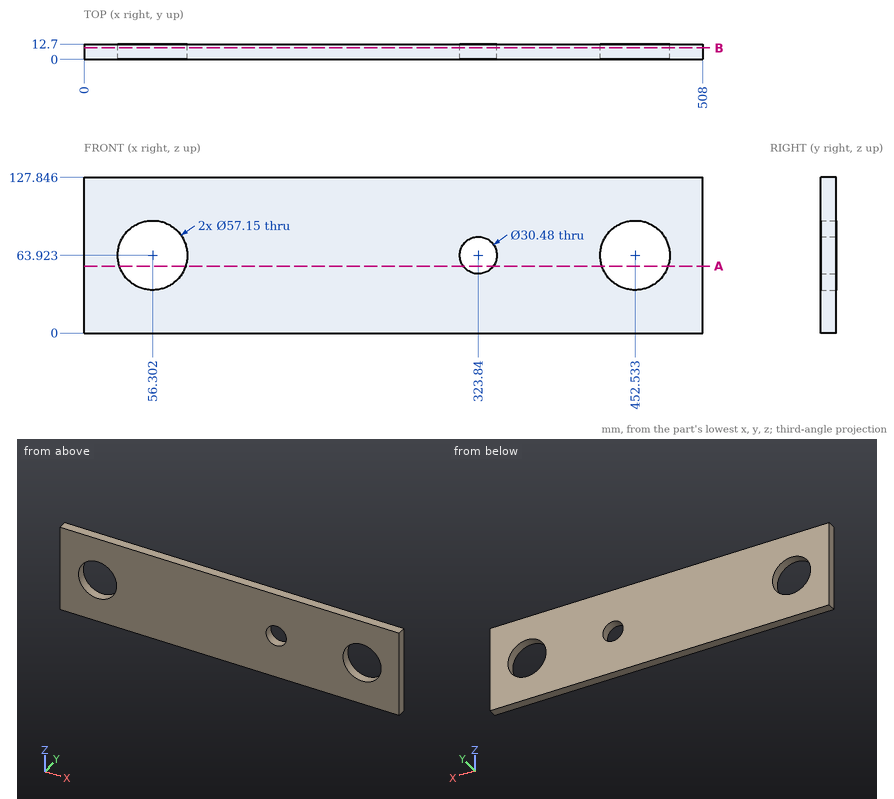
Can you work these out from the drawing? Everything is in mm from the part's minimum corner. Give positions to 0.01 mm unless a question says otherwise; leave off trailing zeros. Order: outer loops, then holes, each group sorted by start corner. A loop starts at its lowest first (then second) coordinate and runs counter-clockwise, first axis right, second up. Notation, with made-up numbers: M -32.75,-39.75 L 15.25,-39.75 A29 cw 15.25,-13.75 Z; hole C 50.25,-36.75 d3. An arc over 180 degrees is marked long. Use a Markdown table: item, result. Add a question column.
Item 1: Suppose I cut it at B-B (y = 9.5). Count the separate pieces of the cut face and the enclosed holes in it, then the cut area to 3 significant figures.
Item 2: If I drill on L1, parallel to X at y = 10.25, z = 60.5; L2, parallel to X at y = 10.75, z = 66; L3, parallel to X at y = 5.75, z = 79.5 (1 decimal), over which ranges is the centre line in solid material (lowest first)? Write a range as [from, to].
Item 3: Suppose I cut it at A-A (z = 55). List the corners of the cut face in (x, y) for me (1 decimal).
Answer sheet:
| question | item | result |
|---|---|---|
| 1 | separate pieces | 1 |
| 1 | enclosed holes | 3 |
| 1 | area | 59,100 mm² |
| 2 | L1 | x = [0, 27.93], [84.67, 308.99], [338.69, 424.16], [480.9, 508] |
| 2 | L2 | x = [0, 27.8], [84.8, 308.74], [338.94, 424.03], [481.03, 508] |
| 2 | L3 | x = [0, 32.3], [80.3, 428.6], [476.5, 508] |
| 3 | outline | M 0,0 L 29.2,0 L 29.2,12.7 L 0,12.7 Z; M 83.4,0 L 311.5,0 L 311.5,12.7 L 83.4,12.7 Z; M 336.2,0 L 425.4,0 L 425.4,12.7 L 336.2,12.7 Z; M 479.7,0 L 508,0 L 508,12.7 L 479.7,12.7 Z |
